Can you work these out from the model? Positions are in its coordinate system, mm. Face numbers are marked on the shaded views. A direction names the side the tool comes from. Give positions to 0.01 mm unless a question says otherwise; leave off trailing zeros. Write each loop counter-clockwise with the first axis right and the second up, starting at its lowest first coordinate (ties: lowest second). Pieces come first, ordered by that corner, then holes.
1. I'm going to push flat-ended pins straight in: pin 1 (1.4 mm diameter, centred on x = 3.5, z = -33, fed in from +Y); pin 2 (4 mm diameter, centred on y = 28, z = -22.5, fed in from -X); pin 3 (3 mm diameter, centred on x = 16.5, z = -24.5, fed in from +Y). Where does each tip first touch, or does it pass through?
2. Suppose I cut it at A-A (y = 35.6). Please give me the cut outline in (x, z).
3. Thinking about a two-plate mould opening in X: for the marked faces 1, 2, 3 and 4, which applies, pulls with the +X half, pulls with the -X half, needs draft (parallel to the pull), parting line crosses it, or undercut?
4. Suppose I cut it at C-C (y = 15). Please give me the cut outline in (x, z).
5. Suppose I cut it at D-D (z = -21.5). Please give me the cut outline in (x, y), and give its area (3 significant figures).
6. On a 3-axis mill with a long thin cutter (end or side, diameter ignored), from which of +Z, -Z, +X, -X, +Y, -Y can I reach the whole of each face in a straight line? I mean the marked faces 5, 6 and 7. Say none if no direction works.
7. If I drill on probe 1 along Y at (x, z) = (38.75, -30.6); probe 2 along Z at (x, y) = (26.5, 3.9) (3 decimals); probe 3 along X at (y, z) = (11, -25.5), over which ranges is the centre line in solid material (lowest first)?
8. Suppose I cut it at B-B (x = 18). Please give me the cut outline in (y, z), and give its area (3 significant figures).
```python
from build123d import *

# Parameters (mm, degrees)
SKETCH1_W                      = 39
SKETCH1_H                      = 35.2
BOSS_EXTRUDE1_DEPTH            = 5
SKETCH2_W                      = 8
SKETCH2_H                      = 35.2
BOSS_EXTRUDE2_DEPTH            = 35.2
SKETCH3_W                      = 4
SKETCH3_H                      = 35.2
BOSS_EXTRUDE3_DEPTH            = 35.2
CUT_EXTRUDE2_REACH             = 41
SKETCH5_R                      = 13
CBORE_FOR_M3_SHCS1_D           = 3.4
CBORE_FOR_M3_SHCS1_DEPTH       = 5
CBORE_FOR_M3_SHCS1_CBORE_D     = 6.5
CBORE_FOR_M3_SHCS1_CBORE_DEPTH = 3
CUT_EXTRUDE3_DEPTH             = 17.6
SKETCH13_R                     = 3
CUT_EXTRUDE5_DEPTH             = 5
SKETCH14_R                     = 11.5
CUT_EXTRUDE6_DEPTH             = 2
CBORE_FOR_M3_SHCS2_D           = 3.4
CBORE_FOR_M3_SHCS2_DEPTH       = 4
CBORE_FOR_M3_SHCS2_CBORE_D     = 6.5
CBORE_FOR_M3_SHCS2_CBORE_DEPTH = 1
SKETCH17_W                     = 8
SKETCH17_H                     = 35.2
CUT_EXTRUDE7_DEPTH             = 17.6


with BuildPart() as part:
    # Sketch1 → Boss-Extrude1 (new body)
    with BuildSketch(Plane(origin=(0, 0, 0), x_dir=(1, 0, 0), z_dir=(0, 1, 0))):
        with Locations((19.5, 17.6)):
            Rectangle(SKETCH1_W, SKETCH1_H)
    extrude(amount=BOSS_EXTRUDE1_DEPTH)

    # Sketch2 → Boss-Extrude2 (add)
    with BuildSketch(Plane(origin=(0, 5, 0), x_dir=(1, 0, 0), z_dir=(0, 1, 0))):
        with Locations((4, 17.6)):
            Rectangle(SKETCH2_W, SKETCH2_H)
    extrude(amount=BOSS_EXTRUDE2_DEPTH)

    # Sketch3 → Boss-Extrude3 (add)
    with BuildSketch(Plane(origin=(0, 5, 0), x_dir=(1, 0, 0), z_dir=(0, 1, 0))):
        with Locations((37, 17.6)):
            Rectangle(SKETCH3_W, SKETCH3_H)
    extrude(amount=BOSS_EXTRUDE3_DEPTH)

    # Sketch5 → Cut-Extrude2 (cut, up to next)
    with BuildSketch(Plane.ZY, mode=Mode.PRIVATE) as cut_extrude2_sk1:
        with Locations((-17.6, 22.6)):
            Circle(SKETCH5_R)
    cut_extrude2_tool1 = extrude(cut_extrude2_sk1.sketch, amount=-CUT_EXTRUDE2_REACH, mode=Mode.PRIVATE) & part.part
    add(cut_extrude2_tool1.solids().sort_by_distance((0, 22.6, -17.6))[0], mode=Mode.SUBTRACT)

    # CBORE for M3 SHCS1
    with Locations(Plane(origin=(0, 5, 0), x_dir=(1, 0, 0), z_dir=(0, 1, 0))):
        with Locations((17.506975999, 13.145005862), (17.500112517, 22.145003245), (26.5, 22.1), (26.5, 13.145005862)):
            CounterBoreHole(CBORE_FOR_M3_SHCS1_D / 2, CBORE_FOR_M3_SHCS1_CBORE_D / 2, CBORE_FOR_M3_SHCS1_CBORE_DEPTH, depth=CBORE_FOR_M3_SHCS1_DEPTH)

    # Sketch10 → Cut-Extrude3 (cut)
    with BuildSketch(Plane(origin=(0, 40.2, 0), x_dir=(1, 0, 0), z_dir=(0, 1, 0))):
        Polygon((37, 20.6), (39, 20.6), (39, 14.6), (37, 14.6), (37, 6.1), (35, 6.1), (35, 29.1), (37, 29.1), align=None)
    extrude(amount=-CUT_EXTRUDE3_DEPTH, mode=Mode.SUBTRACT)

    # Sketch13 → Cut-Extrude5 (cut, through all)
    with BuildSketch(Plane.ZY.offset(-35)):
        with Locations((-17.6, 22.6)):
            Circle(SKETCH13_R)
    extrude(amount=-CUT_EXTRUDE5_DEPTH, mode=Mode.SUBTRACT)

    # Sketch14 → Cut-Extrude6 (cut)
    with BuildSketch(Plane.ZY.offset(-35)):
        with Locations((-17.6, 22.6)):
            Circle(SKETCH14_R)
    extrude(amount=-CUT_EXTRUDE6_DEPTH, mode=Mode.SUBTRACT)

    # CBORE for M3 SHCS2
    with Locations(Plane(origin=(39, 0, 0), x_dir=(0, 0, -1), z_dir=(1, 0, 0))):
        with Locations((30.6, 35.6), (30.6, 9.6), (4.6, 9.6), (4.6, 35.6)):
            CounterBoreHole(CBORE_FOR_M3_SHCS2_D / 2, CBORE_FOR_M3_SHCS2_CBORE_D / 2, CBORE_FOR_M3_SHCS2_CBORE_DEPTH, depth=CBORE_FOR_M3_SHCS2_DEPTH)

    # Sketch17 → Cut-Extrude7 (cut)
    with BuildSketch(Plane(origin=(0, 40.2, 0), x_dir=(1, 0, 0), z_dir=(0, 1, 0))):
        with Locations((4, 17.6)):
            Rectangle(SKETCH17_W, SKETCH17_H)
    extrude(amount=-CUT_EXTRUDE7_DEPTH, mode=Mode.SUBTRACT)


solid = part.part
```
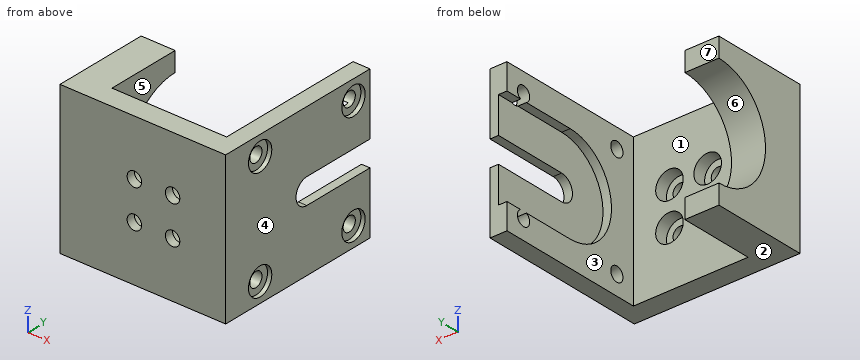
Checks:
1. pin 1: stops at y = 22.6
1. pin 2: stops at x = 37
1. pin 3: stops at y = 5
2. outline: (35, -35.2) - (39, -35.2) - (39, -33.85) - (38, -33.85) - (38, -32.3) - (35, -32.3) - close; (35, -2.9) - (38, -2.9) - (38, -1.35) - (39, -1.35) - (39, 0) - (35, 0) - close; (37, -28.9) - (38, -28.9) - (38, -27.35) - (39, -27.35) - (39, -20.6) - (37, -20.6) - close; (37, -14.6) - (39, -14.6) - (39, -7.85) - (38, -7.85) - (38, -6.3) - (37, -6.3) - close
3. face 1: undercut
3. face 2: needs draft
3. face 3: undercut
3. face 4: pulls with the +X half
4. outline: (0, -35.2) - (8, -35.2) - (8, -28.15) - (0, -28.15) - close; (0, -7.05) - (8, -7.05) - (8, 0) - (0, 0) - close; (35, -35.2) - (39, -35.2) - (39, 0) - (35, 0) - (35, -8.97) - (37, -8.97) - (37, -26.23) - (35, -26.23) - close
5. outline: (0, 0) - (15.93, 0) - (15.93, 2) - (14.31, 2) - (14.31, 5) - (8, 5) - (8, 10.2) - (0, 10.2) - close; (19.07, 0) - (24.91, 0) - (24.91, 2) - (23.31, 2) - (23.31, 5) - (20.69, 5) - (20.69, 2) - (19.07, 2) - close; (28.09, 0) - (39, 0) - (39, 40.2) - (37, 40.2) - (37, 11.78) - (35, 11.78) - (35, 5) - (29.69, 5) - (29.69, 2) - (28.09, 2) - close
5. area: 270 mm2
6. face 5: +Z, -Z, +Y
6. face 6: -X, +Y
6. face 7: +Z, -Z, -X, +Y
7. probe 1: y = 0 to 6.35, 12.85 to 32.35, 38.85 to 40.2
7. probe 2: z = -35.2 to -25.35, -18.85 to -16.395, -9.895 to 0
7. probe 3: x = 0 to 8, 35 to 39
8. outline: (0, -35.2) - (5, -35.2) - (5, -25.36) - (2, -25.36) - (2, -23.77) - (0, -23.77) - close; (0, -20.52) - (2, -20.52) - (2, -18.93) - (5, -18.93) - (5, -16.36) - (2, -16.36) - (2, -14.77) - (0, -14.77) - close; (0, -11.52) - (2, -11.52) - (2, -9.93) - (5, -9.93) - (5, 0) - (0, 0) - close
8. area: 124 mm2
